The listing builds one solid part. Answer for the finished solid, in the listing's coordinates (mm). Face numbers are marked on the shaded views. A direction names the side the tool comes from. Give positions to 0.01 mm unless a question says otherwise; leave off trailing zeros. Loops run counter-clockwise (first coordinate to the right, second up) from the corner with the lowest first, then second, coordinate; pieces in that order, holes last. Notation, with made-up numbers: M 21.25,24.5 L 74.25,24.5 A8 ccw 74.25,35.5 Z; hole C 24,64.5 d6. An arc over 180 degrees is marked long. One line per item, written item: value. Start each with the question number.
Q1. A cutting plane is placed at A-A, the plane z = 50.8. Determine the outline of the cut face in (x, y), and give its area (3 significant figures).
Q2. A cutting plane is placed at C-C, the plane z = 8. Determine the outline of the cut face in (x, y).
Q3. A cutting plane is placed at D-D, the plane x = 30. Determine the outline of the cut face in (y, z), and give its area (3 significant figures).
Q4. For the marked faces 1 and 2, determine the directions among +Z, -Z, +X, -X, +Y, -Y from which every point of the face is accessible in a straight line to the end or side of a thin tool.
Q5. A cutting plane is placed at B-B, the plane y = -18.5. Determine the outline of the cut face in (x, z), and give its area (3 significant figures).
Q6. Consider L1, parallel to X at y = -23.75, z = 19.5; L2, parallel to Y at x = 8, z = 28. Determine where each line is inside the solid, lowest interval first.
Q7. A flat-ended cylindrical pin translates along its axis: pin 1 (5 mm diameter, centred on x = 16.59, z = 50.8, fed in from -Y). Find the tip coordinate at first contact, or state that the pin passes through.
from build123d import *

# Parameters (mm, degrees)
F0_W     = 101.6
F0_H     = 25.4
F0_W_2   = 50.8
F0_H_2   = 12.7
F1_DEPTH = 101.6
F3_DEPTH = 101.601
F5_D     = 6.35


with BuildPart() as f1:
    # F0 (on Top) → F1 (new body)
    with BuildSketch(Plane.XY):
        with Locations((16.590777, -19.253528)):
            Rectangle(F0_W, F0_H)
        with Locations((16.590777, -19.253528)):
            Rectangle(F0_W_2, F0_H_2, mode=Mode.SUBTRACT)
    extrude(amount=F1_DEPTH)

    # F2 (on face) → F3 (cut, through all)
    with BuildSketch(Plane.XY.offset(101.6)):
        Polygon((41.990777, -25.603528), (-8.809223, -25.603528), (-34.209223, -25.603528), (-34.209223, -31.953528), (67.390777, -31.953528), (67.390777, -25.603528), align=None)
    extrude(amount=-F3_DEPTH, mode=Mode.SUBTRACT)

    # F5 (through all)
    with Locations(Plane(origin=(0, -6.553528, 0), x_dir=(-1, 0, 0), z_dir=(0, 1, 0))):
        with Locations((-16.590777, 50.8)):
            Hole(F5_D / 2)


solid = f1.part
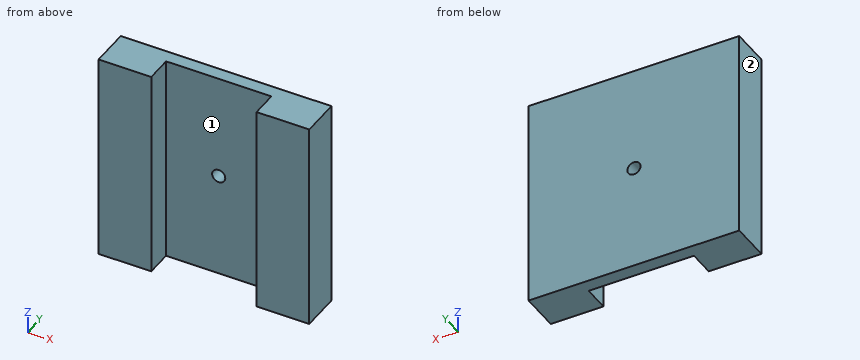
Answer block:
1. outline: M -34.21,-25.6 L -8.81,-25.6 L -8.81,-12.9 L 13.42,-12.9 L 13.42,-6.55 L -34.21,-6.55 Z; M 19.77,-12.9 L 41.99,-12.9 L 41.99,-25.6 L 67.39,-25.6 L 67.39,-6.55 L 19.77,-6.55 Z
1. area: 1,250 mm^2
2. outline: M -34.21,-25.6 L -8.81,-25.6 L -8.81,-12.9 L 41.99,-12.9 L 41.99,-25.6 L 67.39,-25.6 L 67.39,-6.55 L -34.21,-6.55 Z
3. outline: M -12.9,0 L -6.55,0 L -6.55,101.6 L -12.9,101.6 Z
3. area: 645 mm^2
4. face 1: +Z, -Z, -Y
4. face 2: +Z, -Z, -X, +Y, -Y
5. outline: M -34.21,0 L -8.81,0 L -8.81,101.6 L -34.21,101.6 Z; M 41.99,0 L 67.39,0 L 67.39,101.6 L 41.99,101.6 Z
5. area: 5,160 mm^2
6. L1: -34.21 to -8.81, 41.99 to 67.39
6. L2: -12.9 to -6.55
7. pin 1: through
